from build123d import *

# Parameters (mm, degrees)
F0_R     = 3.5
F0_R_2   = 11
F0_R_3   = 2
F1_DEPTH = 10


with BuildPart() as f1:
    # F0 (on Front) → F1 (new body)
    with BuildSketch(Plane.XZ):
        with BuildLine():
            ThreePointArc((90, 140), (87.071068, 147.071068), (80, 150))
            Line((80, 150), (-80, 150))
            ThreePointArc((-80, 150), (-87.071068, 147.071068), (-90, 140))
            Line((-90, 140), (-90, -60))
            ThreePointArc((-90, -60), (-63.63961, -123.63961), (0, -150))
            ThreePointArc((0, -150), (63.63961, -123.63961), (90, -60))
            Line((90, -60), (90, 140))
        make_face()
        with Locations((-80, -60)):
            Circle(F0_R, mode=Mode.SUBTRACT)
        with Locations((0, -60)):
            Circle(F0_R_2, mode=Mode.SUBTRACT)
        with Locations((80, -60)):
            Circle(F0_R, mode=Mode.SUBTRACT)
        with Locations((-80, 140)):
            Circle(F0_R, mode=Mode.SUBTRACT)
        with Locations((-15.5, 84)):
            Circle(F0_R_3, mode=Mode.SUBTRACT)
        with Locations((-15.5, 115)):
            Circle(F0_R_3, mode=Mode.SUBTRACT)
        with Locations((15.5, 84)):
            Circle(F0_R_3, mode=Mode.SUBTRACT)
        with Locations((0, 99.5)):
            Circle(F0_R_2, mode=Mode.SUBTRACT)
        with Locations((15.5, 115)):
            Circle(F0_R_3, mode=Mode.SUBTRACT)
        with Locations((80, 140)):
            Circle(F0_R, mode=Mode.SUBTRACT)
    extrude(amount=F1_DEPTH)


solid = f1.part
Part model, mm, in its own coordinate system. Coordinates: 2 decimals unless noted, no trailing zeros. Loops run counter-clockwise (first coordinate to the right, second up) from the corner with the lowest first, then second, coordinate; pieces in that order, holes last. Notation, with made-up numbers: M 51,28 L 62,28 A16 ccw 62,47 Z; hole C -31.75,89.25 d1. An arc over 180 degrees is marked long. Use a Markdown table: item, result. Add a question column.
Q1. Cut at B-B (x = -37.5). Write the cut outline in (y, z).
Q2. Cut at A-A (y = -5). Give the number of separate pieces and of enclosed holes in the cut face, and give its area (3 significant figures).
Q3. Pin check, flat tips, straight feed: P1, Ø9, axis at x = 80, z = 140, coming from the +Y side; P2, Ø4, axis at x = -80, z = -60, coming from the -Y side; P3, Ø2, axis at y = -4.5, z = -118.5, coming from the -X side; P4, Ø1, axis at x = 4.5, y = -2, coming from the -Z side. Stop position of each tip, or through.
Q4. Cut at C-C (z = -99.5). Write the cut outline in (x, y).
Q5. Probe L1, parallel to X at y = -2.75, z = 140; L2, parallel to Z at x = -80, y = -7; L3, parallel to Z at x = -1, y = -1. List the from-to ranges inside material, lowest first.
Q6. Mould opens along Z. For faces 1 (the flat face through (90, -5, 39)), 2 (the cylindrical face through (87.15, -4.93, 146.99)), 3 (the cylindrical face through (-76.767, -4.93, -61.341)) say: +Z half, -Z half, draft (parallel to the pull), parting line (faces both ways), or undercut.
Worked out:
| question | item | result |
|---|---|---|
| 1 | outline | M -10,-141.82 L 0,-141.82 L 0,150 L -10,150 Z |
| 2 | separate pieces | 1 |
| 2 | enclosed holes | 10 |
| 2 | area | 49,500 mm2 |
| 3 | P1 | stops at y = 0 |
| 3 | P2 | passes through |
| 3 | P3 | stops at x = -69.24 |
| 3 | P4 | stops at z = -149.91 |
| 4 | outline | M -80.87,-10 L 80.87,-10 L 80.87,0 L -80.87,0 Z |
| 5 | L1 | x = -90 to -83.5, -76.5 to 76.5, 83.5 to 90 |
| 5 | L2 | z = -101.23 to -63.5, -56.5 to 136.5, 143.5 to 150 |
| 5 | L3 | z = -149.99 to -70.95, -49.05 to 88.55, 110.45 to 150 |
| 6 | face 1 | draft |
| 6 | face 2 | +Z half |
| 6 | face 3 | undercut |
